from build123d import *

# Parameters (mm, degrees)
SKETCH1_R           = 4
BOSS_EXTRUDE1_DEPTH = 3
SKETCH2_R           = 2.15
BOSS_EXTRUDE2_DEPTH = 4.6
SKETCH3_R           = 1.35
CUT_EXTRUDE1_DEPTH  = 10.474175426
CHAMFER1_SIZE       = 1


with BuildPart() as part:
    # Sketch1 → Boss-Extrude1 (new body)
    with BuildSketch(Plane.XY):
        Circle(SKETCH1_R)
    extrude(amount=BOSS_EXTRUDE1_DEPTH)

    # Sketch2 → Boss-Extrude2 (add)
    with BuildSketch(Plane.XY.offset(3)):
        Circle(SKETCH2_R)
    extrude(amount=BOSS_EXTRUDE2_DEPTH)

    # Sketch3 → Cut-Extrude1 (cut, through all)
    with BuildSketch(Plane.XY.offset(7.6)):
        Circle(SKETCH3_R)
    extrude(amount=-CUT_EXTRUDE1_DEPTH, mode=Mode.SUBTRACT)

    # Chamfer1
    chamfer1_edges = [part.edges().sort_by_distance(p)[0] for p in [
        (-4, 0, 0),
    ]]
    chamfer(chamfer1_edges, length=CHAMFER1_SIZE)


solid = part.part
Input: part model. Units: mm. Frame: model coordinates. A direction names the side the tool comes from. Coordinates: 2 decimals unless noted, no trailing zeros. Loops run counter-clockwise (first coordinate to the right, second up) from the corner with the lowest first, then second, coordinate; pieces in that order, holes last. Notation, with made-up numbers: (-21, 70.5) - (-8, 70.5) arc R19 ccw to (-8, 93.5) - close; hole circle Ø4 at (85, 47.5). An arc over 180 degrees is marked (long way). Answer in a Markdown table with one row per item. Add a question column.
Item 1: Section query C-C on z = 2. Return the cut outline in (x, y).
Item 2: Line query: line 1 along Y through (x, z) = (0, 3.25); line 2 along Y through (x, z) = (0, 2.5); line 3 along Z through (x, y) = (2.25, 0). Output: solid intervals per line, ascending. Write a range as [from, to].
Item 3: Contact query for flat-ended pins moving along their axis: P1, Ø3, axis at x = -3, y = 2.5, coming from the +Z side; P2, Ø3, axis at y = 0.5, z = 6.5, coming from the -X side. Output: stop coordinate, or through.
Item 4: Section query A-A on x = 0. Return the cut outline in (y, z), then the cut area to 3 significant figures.
Item 5: Access query for faces 1 (the flat face through (2, -2, 3)), 2 (the cylindrical face through (-0.29, -1.32, 3.85)). Directions: +Z, -Z, +X, -X, +Y, -Y. A direction counts if a zero-diameter tool reaches every point of the face in a straight line with its end or side. Return the directions, or none.
Item 6: Section query D-D on z = 7.25. Return the cut outline in (x, y).
Recorded:
| question | item | result |
|---|---|---|
| 1 | outline | circle Ø8 at (0, 0); hole circle Ø2.7 at (0, 0) |
| 2 | line 1 | [-2.15, -1.35], [1.35, 2.15] |
| 2 | line 2 | [-4, -1.35], [1.35, 4] |
| 2 | line 3 | [0, 3] |
| 3 | P1 | z = 3 |
| 3 | P2 | x = -2.15 |
| 4 | outline | (-4, 1) - (-3, 0) - (-1.35, 0) - (-1.35, 7.6) - (-2.15, 7.6) - (-2.15, 3) - (-4, 3) - close; (1.35, 0) - (3, 0) - (4, 1) - (4, 3) - (2.15, 3) - (2.15, 7.6) - (1.35, 7.6) - close |
| 4 | area | 22.3 mm^2 |
| 5 | face 1 | +Z |
| 5 | face 2 | +Z, -Z |
| 6 | outline | circle Ø4.3 at (0, 0); hole circle Ø2.7 at (0, 0) |
